Here's how the part is built. I have some questions about the finished solid (model axes, mm). A direction names the side the tool comes from. Give positions to 0.01 mm unless a question says otherwise; leave off trailing zeros. Loops run counter-clockwise (first coordinate to the right, second up) from the corner with the lowest first, then second, coordinate; pieces in that order, holes last. Notation, with made-up numbers: M 18.25,89 L 35.25,89 A34 cw 35.25,119 Z; hole C -39.5,49 d7. An arc over 180 degrees is marked long. Answer as CSV lines item,"result". Start each with the question number.
Item 1: I want a section at A-A on z = 59. List the corners of the cut face in (x, y) for me.
Item 2: I want a section at B-B on x = 80. List the corners of the cut face in (y, z) for me, plus the area to 3 significant figures.
Item 3: If we mould it in two halves opening along X, with no side actions, what happens to faces 4 (the flat face through (48.07, -20.6, 8.67)), 5 (the flat face through (50, -100, 101.6)), 6 (the flat face through (0, -100, 50))? For each: released by +X, released by -X, zero draft, split by the parting line, or undercut.
Item 4: If I drill on line 1 along X through (y, z) = (-98, 69); line 2 along Y through (x, z) = (82, 61.5), over which ranges is the centre line in solid material (lowest first)? Write a range as from..to.
Item 5: For faces 1 (the flat face through (48.07, -20.6, 92.93)), 2 (the flat face through (76.2, -105, 66)), 3 (the flat face through (101.6, -100, 50)), which set-ups out of +Z, -Z, +X, -X, +Y, -Y let a thin tool reach every point of the face, with its end or its side?
from build123d import *

# Parameters (mm, degrees)
F0_W          = 101.6
F0_H          = 101.6
F1_DEPTH      = 203.2
F4_R          = 3.175
F5_DEPTH      = 89.8035612107
F4_R_2        = 6.35
F6_DEPTH      = 9.525
F6_DEPTH_BACK = 125.724585695
F8_R          = 14.9564756193
F9_DEPTH      = 25.4


# Not quite as in the source:
# - a pattern or mirror of a feature is missing from the dataset's text; its kind, count and spacing are read off the source's solid


with BuildPart() as f1:
    # F0 (on Front) → F1 (new body)
    with BuildSketch(Plane.XZ):
        with Locations((50.8, 50.8)):
            Rectangle(F0_W, F0_H)
    extrude(amount=F1_DEPTH)

    # F4 (on line) → F5 (cut, through all)
    with BuildSketch(Plane(origin=(0, -63.5, 63.5), x_dir=(-1, 0, 0), z_dir=(0, 0.7071067812, -0.7071067812))):
        with Locations((-50.8, 53.8815367264)):
            Circle(F4_R)
    f5 = extrude(amount=F5_DEPTH, mode=Mode.SUBTRACT)

    # F5_copies: F5 across plane
    add(f5.mirror(Plane(origin=(0, 1.2e-05, 50.799992), x_dir=(-1, 0, 0), z_dir=(0, 0, -1))), mode=Mode.SUBTRACT)

    # F4 (on line) → F6 (cut, two sides)
    with BuildSketch(Plane(origin=(0, -63.5, 63.5), x_dir=(-1, 0, 0), z_dir=(0, 0.7071067812, -0.7071067812))) as f6_sk:
        with Locations((-50.8, 53.8815367264)):
            Circle(F4_R_2)
        with Locations((-50.8, 53.8815367264)):
            Circle(F4_R, mode=Mode.SUBTRACT)
        with Locations((-50.8, 53.8815367264)):
            Circle(F4_R)
    f6 = extrude(amount=F6_DEPTH, mode=Mode.SUBTRACT) + extrude(f6_sk.sketch, amount=-F6_DEPTH_BACK, mode=Mode.SUBTRACT)

    # F6_copies: F6 across plane
    add(f6.mirror(Plane(origin=(0, 2.8e-05, 50.79997), x_dir=(0, -1, 1e-06), z_dir=(0, -1e-06, -1))), mode=Mode.SUBTRACT)

    # F8 (on face) → F9 (cut)
    with BuildSketch(Plane.YZ.offset(101.6)):
        with Locations((-104.4293493032, 65.6716227531)):
            Circle(F8_R)
    extrude(amount=-F9_DEPTH, mode=Mode.SUBTRACT)


solid = f1.part
Result:
1,outline,"M 0,-203.2 L 101.6,-203.2 L 101.6,-117.82 L 76.2,-117.82 L 76.2,-91.04 L 101.6,-91.04 L 101.6,0 L 0,0 Z"
2,outline,"M -203.2,0 L 0,0 L 0,101.6 L -203.2,101.6 Z; hole C -104.43,65.67 d29.91"
2,area,"19,900 mm^2"
3,face 4,"undercut"
3,face 5,"zero draft"
3,face 6,"released by -X"
4,line 1,"0..76.2"
4,line 2,"-203.2..-118.79, -90.07..0"
5,face 1,"none"
5,face 2,"+X"
5,face 3,"+Z, -Z, +X, +Y, -Y"
